Read the model definition and answer for the solid it produces. Units are mm, in the model's axes. Face numbers are marked on the shaded views. A direction names the side the tool comes from. Coordinates: 2 decimals unless noted, no trailing zeros. Write each loop counter-clockwise with the first axis right and the second up, starting at its lowest first coordinate (ties: lowest second). Pieces come first, ordered by that corner, then holes. Notation, with made-up numbers: (-3, 5) - (40, 5) arc R25 cw to (40, 22) - close; hole circle Ø6 at (-35.75, 85). An arc over 180 degrees is marked (long way). Return JSON: item names as keys, results as strings.
```python
from build123d import *

# Parameters (mm, degrees)
F0_W      = 134.2095732689
F0_H      = 54.8827461898
F1_DEPTH  = 25.4
F2_R      = 16.9227775992
F3_DEPTH  = 62.23
F4_R      = 29.2955411645
F5_DEPTH  = 59.944
F6_DEPTH  = 46.482
F8_W      = 25.8811749518
F8_H      = 28.2603334635
F9_DEPTH  = 153.162
F11_R     = 25.1124764346
F12_DEPTH = 90.932
F13_DEPTH = 104.648


with BuildPart() as f1:
    # F0 (on Right) → F1 (new body)
    with BuildSketch(Plane.YZ):
        Polygon((-81.9051712751, -7.1336217225), (-81.9051712751, 47.7491244674), (-142.8231298923, 47.7491244674), (-165.6134873629, 11.0719772056), (-172.7062016726, -51.1080250144), (-149.0172445774, -75.3351673484), (-108.8246330619, -75.3351673484), align=None)
        with Locations((-14.8003846407, 20.3077513725)):
            Rectangle(F0_W, F0_H)
    extrude(amount=F1_DEPTH)

    # F2 (on face) → F3 (join)
    with BuildSketch(Plane(origin=(0, 52.3044019938, 0), x_dir=(-1, 0, 0), z_dir=(0, 1, 0))):
        with Locations((-12.7, 20.3077513725)):
            Circle(F2_R)
    extrude(amount=F3_DEPTH)

    # F4 (on face) → F5 (join)
    with BuildSketch(Plane(origin=(0, 114.5344019938, 0), x_dir=(-1, 0, 0), z_dir=(0, 1, 0))):
        with Locations((-12.7, 20.3077513725)):
            Circle(F4_R)
    extrude(amount=F5_DEPTH)

    # F0 (on Right) → F6 (join)
    with BuildSketch(Plane.YZ):
        Polygon((-81.9051712751, -7.1336217225), (-81.9051712751, 47.7491244674), (-142.8231298923, 47.7491244674), (-165.6134873629, 11.0719772056), (-172.7062016726, -51.1080250144), (-149.0172445774, -75.3351673484), (-108.8246330619, -75.3351673484), align=None)
        with Locations((-14.8003846407, 20.3077513725)):
            Rectangle(F0_W, F0_H)
    extrude(amount=F6_DEPTH)

    # F8 (on face) → F9 (join)
    with BuildSketch(Plane(origin=(0, 0, -7.1336217225), x_dir=(1, 0, 0), z_dir=(0, 0, -1))):
        with Locations((12.9405874759, -3.3692447469)):
            Rectangle(F8_W, F8_H)
    extrude(amount=F9_DEPTH)

    # F11 (on face) → F12 (join)
    with BuildSketch(Plane(origin=(0, 174.4784019938, 0), x_dir=(-1, 0, 0), z_dir=(0, 1, 0))):
        with Locations((-11.6089172661, 17.1811357141)):
            Circle(F11_R)
    extrude(amount=F12_DEPTH)

    # F13 (add): a face of the model
    f13_faces = [f1.faces().sort_by_distance(p)[0] for p in [
        (23.241, -128.9209388196, -75.3351673484),
    ]]
    extrude(f13_faces, amount=F13_DEPTH)


solid = f1.part
```
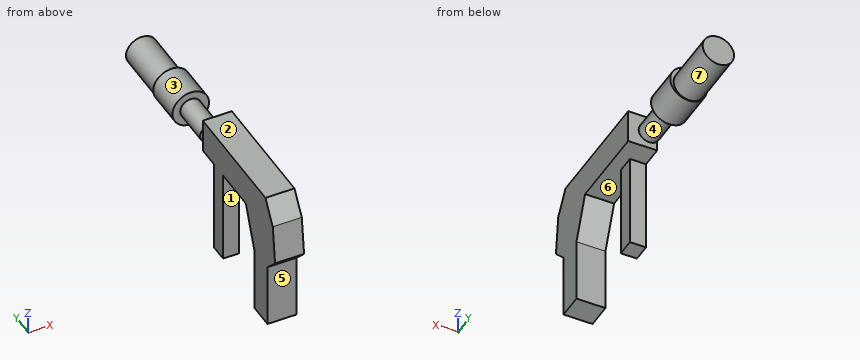
(1) Flat-ended cylindrical pins translate along their axes: P1, Ø8, axis at x = 14, z = -93, coming from the -Y side; P2, Ø14, axis at x = 34, y = -66, coming from the +Z side; P3, Ø17.5, axis at x = 9, z = 25, coming from the -Y side. Find the tip coordinate at first contact, or state that the pin passes through.
Answer:
{"P1": "y = -149.02", "P2": "z = 47.75", "P3": "y = -162.4"}
(2) A cutting plane is placed at D-D (y = 208.5). Determine the outline of the cut face in (x, z), and give its area (3 significant figures).
Answer:
{"outline": "circle Ø50.22 at (11.61, 17.18)", "area": "1,980 mm²"}
(3) A cutting plane is placed at B-B (y = -138.5). Determine the outline of the cut face in (x, z).
Answer:
{"outline": "(0, -179.98) - (46.48, -179.98) - (46.48, 47.75) - (0, 47.75) - close"}
(4) A cutting plane is placed at A-A (x = 15). Determine the outline of the cut face in (y, z), and give its area (3 significant figures).
Answer:
{"outline": "(-172.71, -51.11) - (-149.02, -75.34) - (-149.02, -179.98) - (-108.82, -179.98) - (-108.82, -75.34) - (-81.91, -7.13) - (-10.76, -7.13) - (-10.76, -160.3) - (17.5, -160.3) - (17.5, -7.13) - (52.3, -7.13) - (52.3, 3.54) - (114.53, 3.54) - (114.53, -8.9) - (174.48, -8.9) - (174.48, -7.7) - (265.41, -7.7) - (265.41, 42.06) - (174.48, 42.06) - (174.48, 49.51) - (114.53, 49.51) - (114.53, 37.07) - (52.3, 37.07) - (52.3, 47.75) - (-142.82, 47.75) - (-165.61, 11.07) - close", "area": "35,100 mm²"}
(5) Straight lines are drawn through the part: line 1 (Y direction, x = 24.5, z = -88); line 2 (X direction, y = 14, z = -10.5); line 3 (Y direction, x = 8.5, z = -23). For each, find the intervals that lie inside material, in ascending order. Write a range as from..to.
Answer:
{"line 1": "-149.02..-108.82, -10.76..17.5", "line 2": "0..25.88", "line 3": "-169.5..-88.17, -10.76..17.5"}
(6) Determine the mould class of the marked faces 5, 6 and 7 for opening direction Y: +Y half, -Y half, draft (parallel to the pull), parting line (faces both ways), or undercut.
Answer:
{"face 5": "-Y half", "face 6": "undercut", "face 7": "draft"}
(7) Which of the six approach directions +Z, -Z, +X, -X, +Y, -Y give full straight-line access (tool end or side, diameter ignored) to the marked faces 1, 2, 3 and 4?
Answer:
{"face 1": "-Z, +X, -X", "face 2": "+Z, +X, -X, -Y", "face 3": "+Y", "face 4": "none"}
(8) A cutting plane is placed at C-C (y = -58). Determine the outline of the cut face in (x, z).
Answer:
{"outline": "(0, -7.13) - (46.48, -7.13) - (46.48, 47.75) - (0, 47.75) - close"}
